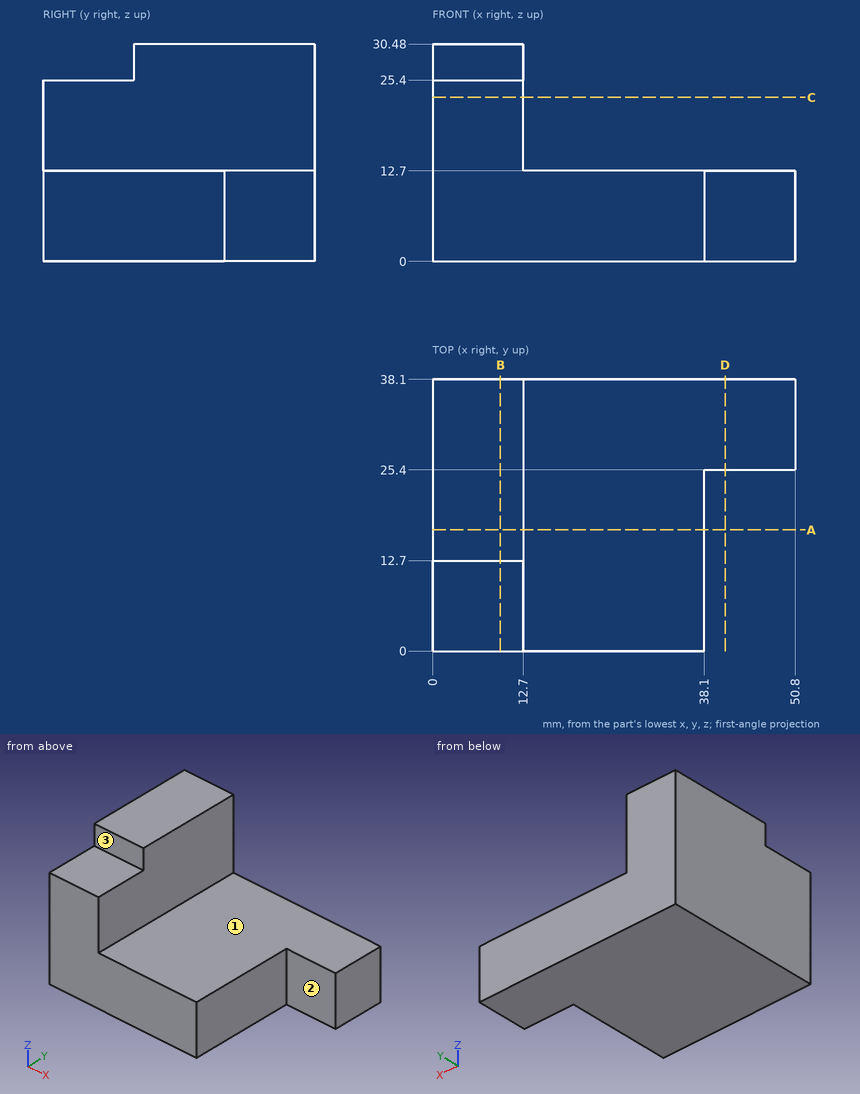
For this review, use the dimensioned drawing (mm, ordinates from the lowest corner) and the shaded views. A direction names the side the tool comes from. Give positions to 0.01 mm unless a question says otherwise; leave off trailing zeros. Write each loop counter-clockwise with the first axis right and the second up, starting at its lowest first coordinate (ties: lowest second). Pieces come first, ordered by that corner, then holes. Notation, with made-up numbers: M 44,10 L 91,10 A13 ccw 91,17 Z; hole C 21.5,83 d9. An arc over 180 degrees is marked long. Write item = value, one per line. Start each with the question number.
Q1. We need section C-C (z = 23). State the section outline as (x, y) points, plus the area to 3 significant figures.
Q2. We need section A-A (y = 17). State the section outline as (x, z) points, plus the area to 3 significant figures.
Q3. We need section B-B (x = 9.5). State the section outline as (y, z) points, plus the area to 3 significant figures.
Q4. For line 1 (Z direction, x = 26, y = 18.5); line 2 (Y direction, x = 49.5, z = 3.5); line 3 (X direction, y = 16, z = 10), list the stretches that pass through material, from the lowest coordinate up.
Q5. Machinability: for the marked faces 1, 2 and 3, which of the approach directions +Z, -Z, +X, -X, +Y, -Y give a long, thin tool a straight path to every point of the face, cutting with its end or side? Answer none if there is none.
Q6. We need section D-D (x = 41). State the section outline as (y, z) points.
Q7. Clearance check with flat-ended pins moving along their axes: pin 1 (5.5 mm diameter, centred on y = 27.5, z = 22, fed in from +X); pin 2 (5 mm diameter, centred on x = 22, y = 18, fed in from +Z); pin 3 (4 mm diameter, centred on y = 11, z = 4.5, fed in from +X). State where each tip first meets the part, or that it passes through.
Result set:
q1.outline = M 0,0 L 12.7,0 L 12.7,38.1 L 0,38.1 Z
q1.area = 484 mm2
q2.outline = M 0,0 L 38.1,0 L 38.1,12.7 L 12.7,12.7 L 12.7,30.48 L 0,30.48 Z
q2.area = 710 mm2
q3.outline = M 0,0 L 38.1,0 L 38.1,30.48 L 12.7,30.48 L 12.7,25.4 L 0,25.4 Z
q3.area = 1,100 mm2
q4.line_1 = 0 to 12.7
q4.line_2 = 25.4 to 38.1
q4.line_3 = 0 to 38.1
q5.face_1 = +Z, +X, +Y, -Y
q5.face_2 = +Z, -Z, +X, -Y
q5.face_3 = +Z, +X, -X, -Y
q6.outline = M 25.4,0 L 38.1,0 L 38.1,12.7 L 25.4,12.7 Z
q7.pin_1 = 12.7
q7.pin_2 = 12.7
q7.pin_3 = 38.1
